Read the model definition and answer for the solid it produces. Units are mm, in the model's axes. A direction names the side the tool comes from. Round coordinates to 2 decimals unless told otherwise and drop trailing zeros. Loops run counter-clockwise (first coordinate to the right, second up) from the corner with the lowest first, then second, coordinate; pieces in that order, holes last. Notation, with made-up numbers: M 75,7.25 L 133,7.25 A18 cw 133,13.25 Z; hole C 77,-21.75 d2. An arc over 180 degrees is marked long. Write each question's results on one line, items separated by ' | '.
```python
from build123d import *

# Parameters (mm, degrees)
SKETCH_1_W          = 28.7
SKETCH_1_H          = 18.2
EXTRUDE_1_DEPTH     = 1
SKETCH_2_R          = 0.925
CUT_EXTRUDE_1_DEPTH = 49.82096668
SKETCH_3_R          = 0.925
SKETCH_3_R_2        = 0.65
EXTRUDE_2_DEPTH     = 0.5


with BuildPart() as part:
    # 草圖1 → 填料-伸長1 (new body)
    with BuildSketch(Plane.XY):
        with Locations((12.170607589, 31.877361563)):
            Rectangle(SKETCH_1_W, SKETCH_1_H)
    extrude(amount=EXTRUDE_1_DEPTH)

    # 草圖2 → 除料-伸長1 (cut, through all)
    with BuildSketch(Plane.XY.offset(1)):
        with Locations((25.570607589, 34.377361563)):
            Circle(SKETCH_2_R)
        with Locations((25.570607589, 29.377361563)):
            Circle(SKETCH_2_R)
        with Locations((-1.229392411, 34.377361563)):
            Circle(SKETCH_2_R)
        with Locations((-1.229392411, 29.377361563)):
            Circle(SKETCH_2_R)
    extrude(amount=-CUT_EXTRUDE_1_DEPTH, mode=Mode.SUBTRACT)

    # 草圖3 → 填料-伸長2 (add)
    # profile 1 of 4: a face of its own
    with BuildSketch(Plane(origin=(0, 0, 1), x_dir=(-1, 0, 0), z_dir=(0, 0, -1))):
        with Locations(Location((1.229392411, 34.377361563, 0), (0, 0, 180))):
            Circle(SKETCH_3_R)
        with Locations(Location((1.229392411, 34.377361563, 0), (0, 0, 90))):
            Circle(SKETCH_3_R_2, mode=Mode.SUBTRACT)
    # profile 2 of 4: a face of its own
    with BuildSketch(Plane(origin=(0, 0, 1), x_dir=(-1, 0, 0), z_dir=(0, 0, -1))):
        with Locations(Location((1.229392411, 29.377361563, 0), (0, 0, 180))):
            Circle(SKETCH_3_R)
        with Locations(Location((1.229392411, 29.377361563, 0), (0, 0, 270))):
            Circle(SKETCH_3_R_2, mode=Mode.SUBTRACT)
    # profile 3 of 4: a face of its own
    with BuildSketch(Plane(origin=(0, 0, 1), x_dir=(-1, 0, 0), z_dir=(0, 0, -1))):
        with Locations(Location((-25.570607589, 29.377361563, 0), (0, 0, 180))):
            Circle(SKETCH_3_R)
        with Locations(Location((-25.570607589, 29.377361563, 0), (0, 0, 90))):
            Circle(SKETCH_3_R_2, mode=Mode.SUBTRACT)
    # profile 4 of 4: a face of its own
    with BuildSketch(Plane(origin=(0, 0, 1), x_dir=(-1, 0, 0), z_dir=(0, 0, -1))):
        with Locations(Location((-25.570607589, 34.377361563, 0), (0, 0, 180))):
            Circle(SKETCH_3_R)
        with Locations(Location((-25.570607589, 34.377361563, 0), (0, 0, 270))):
            Circle(SKETCH_3_R_2, mode=Mode.SUBTRACT)
    extrude(amount=EXTRUDE_2_DEPTH)


solid = part.part
```
1. Determine the mould class of faces 1 (the face through (26.01, 28.9, 0.75)), 2 (the face through (12, 32, 1)), 3 (the face through (26.521, 31.7, 0.5)), 4 (the face through (-2.179, 31.7, 0.5)) for opening direction X: released by +X, released by -X, zero draft, split by the parting line, or undercut.
Completed:
face 1: undercut | face 2: zero draft | face 3: released by +X | face 4: released by -X
2. Find the intervals of material crossed by L1, parallel to X at y = 30, z = 0.15, in increasing order.
Completed:
L1: x = -2.18 to -1.91, -0.55 to 24.89, 26.25 to 26.52
3. Which of the six approach directions +Z, -Z, +X, -X, +Y, -Y give full straight-line access (tool end or side, diameter ignored) to faces 5 (the face through (24.889, 35.003, 0.254)), 6 (the face through (12, 32, 0))?
Completed:
face 5: -Z | face 6: -Z, +X, -X, +Y, -Y
4. Find section A-A, the plane y = 34. Give the vertices of the cut face in (x, z).
Completed:
outline: M -2.18,0 L -2.07,0 L -2.07,0.5 L -1.76,0.5 L -1.76,1 L -2.18,1 Z; M -0.7,0.5 L -0.38,0.5 L -0.38,0 L 24.73,0 L 24.73,0.5 L 25.04,0.5 L 25.04,1 L -0.7,1 Z; M 26.1,0.5 L 26.42,0.5 L 26.42,0 L 26.52,0 L 26.52,1 L 26.1,1 Z
5. Given P1, Ø0.9, axis at x = 25.5, y = 29, coming from the -Z side; P2, Ø0.6, axis at x = -1, y = 34.5, coming from the -Z side, each flat-ended and moving along its own axis, determine where each tip first touches the part or whether it passes through.
Completed:
P1: stops at z = 0.5 | P2: passes through
6. Find section B-B, the plane z = 0.25. Give the vertices of the cut face in (x, y) (3 decimals).
Completed:
outline: M -2.179,22.777 L 26.521,22.777 L 26.521,40.977 L -2.179,40.977 Z; hole C -1.229,29.377 d1.85; hole C -1.229,34.377 d1.85; hole C 25.571,29.377 d1.85; hole C 25.571,34.377 d1.85
